```python
from build123d import *

# Parameters (mm, degrees)
SKETCH_2_W          = 180
SKETCH_2_H          = 180
EXTRUDE_1_DEPTH     = 5
EXTRUDE_1_2_DEPTH   = 115
EXTRUDE_2_DEPTH     = 2
CUT_EXTRUDE_1_DEPTH = 145.5
SKETCH_6_R          = 6.5
CUT_EXTRUDE_2_DEPTH = 6
FILLET_1_R          = 10
CUT_EXTRUDE_3_REACH = 146


with BuildPart() as part:
    # Эскиз2 → Extrude 1 (new body)
    with BuildSketch(Plane(origin=(0, 0, 0), x_dir=(1, 0, 0), z_dir=(0, 1, 0))):
        Rectangle(SKETCH_2_W, SKETCH_2_H)
    extrude(amount=EXTRUDE_1_DEPTH)

    # Эскиз3 → Extrude 1 2 (add)
    with BuildSketch(Plane(origin=(0, 5, 0), x_dir=(1, 0, 0), z_dir=(0, 1, 0))):
        with BuildLine():
            Line((-50.5, -50), (-50.5, 49))
            ThreePointArc((-50.5, 49), (-50.207106781, 49.707106781), (-49.5, 50))
            Line((-49.5, 50), (49.5, 50))
            ThreePointArc((49.5, 50), (50.207106781, 49.707106781), (50.5, 49))
            Line((50.5, 49), (50.5, -50))
            Line((50.5, -50), (54.5, -50))
            Line((54.5, -50), (54.5, 49))
            ThreePointArc((54.5, 49), (53.035533906, 52.535533906), (49.5, 54))
            Line((49.5, 54), (-49.5, 54))
            ThreePointArc((-49.5, 54), (-53.035533906, 52.535533906), (-54.5, 49))
            Line((-54.5, 49), (-54.5, -50))
            Line((-54.5, -50), (-50.5, -50))
        make_face()
    extrude(amount=EXTRUDE_1_2_DEPTH)

    # Эскиз4 → Бобышка-Вытянуть2 (add, symmetric)
    with BuildSketch(Plane(origin=(0, 0, 0), x_dir=(0, 0, -1), z_dir=(1, 0, 0))):
        Polygon((54, 58.693575035), (85, 5), (54, 5), align=None)
    extrude(amount=EXTRUDE_2_DEPTH, both=True)

    # Эскиз5 → Вырез-Вытянуть1 (cut, through all)
    with BuildSketch(Plane(origin=(54.5, 0, 0), x_dir=(0, 0, -1), z_dir=(1, 0, 0))):
        with BuildLine():
            Line((-20, 108), (-20, 96))
            ThreePointArc((-20, 96), (-25, 91), (-30, 96))
            Line((-30, 96), (-30, 108))
            ThreePointArc((-30, 108), (-25, 113), (-20, 108))
        make_face()
        with BuildLine():
            Line((-20, 29), (-20, 17))
            ThreePointArc((-20, 17), (-25, 12), (-30, 17))
            Line((-30, 17), (-30, 29))
            ThreePointArc((-30, 29), (-25, 34), (-20, 29))
        make_face()
        with BuildLine():
            Line((20, 108), (20, 96))
            ThreePointArc((20, 96), (25, 91), (30, 96))
            Line((30, 96), (30, 108))
            ThreePointArc((30, 108), (25, 113), (20, 108))
        make_face()
        with BuildLine():
            Line((20, 29), (20, 17))
            ThreePointArc((20, 17), (25, 12), (30, 17))
            Line((30, 17), (30, 29))
            ThreePointArc((30, 29), (25, 34), (20, 29))
        make_face()
    extrude(amount=-CUT_EXTRUDE_1_DEPTH, mode=Mode.SUBTRACT)

    # Эскиз6 → Вырез-Вытянуть2 (cut, through all)
    with BuildSketch(Plane(origin=(0, 5, 0), x_dir=(1, 0, 0), z_dir=(0, 1, 0))):
        with Locations(Location((-75, 75, 0), (0, 0, 270))):  # turned: the seam where the file's is
            Circle(SKETCH_6_R)
        with Locations(Location((-75, -75, 0), (0, 0, 270))):  # turned: the seam where the file's is
            Circle(SKETCH_6_R)
        with Locations(Location((75, 75, 0), (0, 0, 270))):  # turned: the seam where the file's is
            Circle(SKETCH_6_R)
        with Locations(Location((75, -75, 0), (0, 0, 270))):  # turned: the seam where the file's is
            Circle(SKETCH_6_R)
    extrude(amount=-CUT_EXTRUDE_2_DEPTH, mode=Mode.SUBTRACT)

    # Скругление1
    fillet_1_edges = [part.edges().sort_by_distance(p)[0] for p in [
        (90, 2.5, 90),
        (-90, 2.5, 90),
        (-90, 2.5, -90),
        (90, 2.5, -90),
    ]]
    fillet(fillet_1_edges, radius=FILLET_1_R)

    # Эскиз8 → Вырез-Вытянуть3 (cut, up to next)
    with BuildSketch(Plane(origin=(0, 0, -54), x_dir=(-1, 0, 0), z_dir=(0, 0, -1)), mode=Mode.PRIVATE) as cut_extrude_3_sk1:
        with BuildLine():
            Line((-20, 108), (-20, 96))
            ThreePointArc((-20, 96), (-25, 91), (-30, 96))
            Line((-30, 96), (-30, 108))
            ThreePointArc((-30, 108), (-25, 113), (-20, 108))
        make_face()
    cut_extrude_3_tool1 = extrude(cut_extrude_3_sk1.sketch, amount=-CUT_EXTRUDE_3_REACH, mode=Mode.PRIVATE) & part.part
    add(cut_extrude_3_tool1.solids().sort_by_distance((25, 102, -54))[0], mode=Mode.SUBTRACT)
    # Эскиз8 → Вырез-Вытянуть3 (cut, up to next)
    with BuildSketch(Plane(origin=(0, 0, -54), x_dir=(-1, 0, 0), z_dir=(0, 0, -1)), mode=Mode.PRIVATE) as cut_extrude_3_sk2:
        with BuildLine():
            Line((-20, 29), (-20, 17))
            ThreePointArc((-20, 17), (-25, 12), (-30, 17))
            Line((-30, 17), (-30, 29))
            ThreePointArc((-30, 29), (-25, 34), (-20, 29))
        make_face()
    cut_extrude_3_tool2 = extrude(cut_extrude_3_sk2.sketch, amount=-CUT_EXTRUDE_3_REACH, mode=Mode.PRIVATE) & part.part
    add(cut_extrude_3_tool2.solids().sort_by_distance((25, 23, -54))[0], mode=Mode.SUBTRACT)
    # Эскиз8 → Вырез-Вытянуть3 (cut, up to next)
    with BuildSketch(Plane(origin=(0, 0, -54), x_dir=(-1, 0, 0), z_dir=(0, 0, -1)), mode=Mode.PRIVATE) as cut_extrude_3_sk3:
        with BuildLine():
            Line((20, 108), (20, 96))
            ThreePointArc((20, 96), (25, 91), (30, 96))
            Line((30, 96), (30, 108))
            ThreePointArc((30, 108), (25, 113), (20, 108))
        make_face()
    cut_extrude_3_tool3 = extrude(cut_extrude_3_sk3.sketch, amount=-CUT_EXTRUDE_3_REACH, mode=Mode.PRIVATE) & part.part
    add(cut_extrude_3_tool3.solids().sort_by_distance((-25, 102, -54))[0], mode=Mode.SUBTRACT)
    # Эскиз8 → Вырез-Вытянуть3 (cut, up to next)
    with BuildSketch(Plane(origin=(0, 0, -54), x_dir=(-1, 0, 0), z_dir=(0, 0, -1)), mode=Mode.PRIVATE) as cut_extrude_3_sk4:
        with BuildLine():
            Line((20, 29), (20, 17))
            ThreePointArc((20, 17), (25, 12), (30, 17))
            Line((30, 17), (30, 29))
            ThreePointArc((30, 29), (25, 34), (20, 29))
        make_face()
    cut_extrude_3_tool4 = extrude(cut_extrude_3_sk4.sketch, amount=-CUT_EXTRUDE_3_REACH, mode=Mode.PRIVATE) & part.part
    add(cut_extrude_3_tool4.solids().sort_by_distance((-25, 23, -54))[0], mode=Mode.SUBTRACT)


solid = part.part
```
Could you check a few things on this model? Use its own coordinates, in mm. A direction names the side the tool comes from. Round coordinates to 2 decimals unless told otherwise and drop trailing zeros. Loops run counter-clockwise (first coordinate to the right, second up) from the corner with the lowest first, then second, coordinate; pieces in that order, holes last.
Q1. I want a section at D-D (x = -5). Write out the boundary of the cut face in (y, z).
Q2. I want a section at B-B (z = 75). Write out the boundary of the cut face in (x, y).
Q3. Thinking about a two-plate mould opening in Y: for faces 1 (the cylindrical face through (-52, 34, -25)), 2 (the flat face through (-54.5, 62, 0)), which applies, pulls with the +Y half, pulls with the -Y half, needs draft (parallel to the pull), parting line crosses it, or undercut?
Q4. Please list where these lines run through material, in increasing order: L1, parallel to X at y = 3, z = 75; L2, parallel to X at y = 113, z = -4; L3, parallel to Y at x = 18, z = 34.5.
Q5. On a 3-axis mill with a long thin cutter (end or side, diameter ignored), from which of +Z, -Z, +X, -X, +Y, -Y can I reach the whole of each face in a straight line? I mean faces 3 (the flat face through (54.5, 62, 1)), 4 (the cylindrical face through (53, 12, 25)), 5 (the cylindrical face through (25, 113, -52)). Say none if no direction works.
Q6. For P1, Ø1.2, axis at x = 52, y = 100, coming from the +Z side; P2, Ø2, axis at y = 21, z = -51.5, coming from the +X side; P3, Ø12, axis at x = 4, y = 16, coming from the -Z side, each with a flat end and sliding along its axis, tell me the tip position at first contact or that it passes through.
Q7. I want a section at C-C (z = 25). Write out the boundary of the cut face in (x, y).
Q8. I want a section at A-A (x = 75). Write out the boundary of the cut face in (y, z).
Answer below:
1. outline: (0, -90) - (5, -90) - (5, -54) - (120, -54) - (120, -50) - (5, -50) - (5, 90) - (0, 90) - close
2. outline: (-90, 0) - (-81.5, 0) - (-81.5, 5) - (-90, 5) - close; (-68.5, 0) - (68.5, 0) - (68.5, 5) - (-68.5, 5) - close; (81.5, 0) - (90, 0) - (90, 5) - (81.5, 5) - close
3. face 1: undercut
3. face 2: needs draft
4. L1: x = -90 to -81.5, -68.5 to 68.5, 81.5 to 90
4. L2: x = -54.5 to -50.5, 50.5 to 54.5
4. L3: y = 0 to 5
5. face 3: +Z, -Z, +X, +Y
5. face 4: +X, -X
5. face 5: +Z, -Z
6. P1: stops at z = 50
6. P2: stops at x = 54.27
6. P3: stops at z = -81.92
7. outline: (-90, 0) - (90, 0) - (90, 5) - (54.5, 5) - (54.5, 12) - (50.5, 12) - (50.5, 5) - (-50.5, 5) - (-50.5, 12) - (-54.5, 12) - (-54.5, 5) - (-90, 5) - close; (-54.5, 34) - (-50.5, 34) - (-50.5, 91) - (-54.5, 91) - close; (-54.5, 113) - (-50.5, 113) - (-50.5, 120) - (-54.5, 120) - close; (50.5, 34) - (54.5, 34) - (54.5, 91) - (50.5, 91) - close; (50.5, 113) - (54.5, 113) - (54.5, 120) - (50.5, 120) - close
8. outline: (0, -90) - (5, -90) - (5, -81.5) - (0, -81.5) - close; (0, -68.5) - (5, -68.5) - (5, 68.5) - (0, 68.5) - close; (0, 81.5) - (5, 81.5) - (5, 90) - (0, 90) - close
